from build123d import *

# Parameters (mm, degrees)
CROQUIS5_R              = 10
SALIENTE_EXTRUIR1_DEPTH = 9
CROQUIS6_R              = 14.5
SALIENTE_EXTRUIR2_DEPTH = 13
CROQUIS7_R              = 22
SALIENTE_EXTRUIR3_DEPTH = 6
CROQUIS8_R              = 12
CORTAR_EXTRUIR1_DEPTH   = 16
CROQUIS9_R              = 3
CORTAR_EXTRUIR2_DEPTH   = 16
CROQUIS10_W             = 3
CROQUIS10_H             = 9
SALIENTE_EXTRUIR4_DEPTH = 13
SALIENTE_EXTRUIR5_DEPTH = 13
CROQUIS12_W             = 8
CROQUIS12_H             = 3.8
CORTAR_EXTRUIR3_DEPTH   = 13
CROQUIS13_R             = 3
CORTAR_EXTRUIR4_DEPTH   = 13
CROQUIS14_R             = 2.05
CORTAR_EXTRUIR5_DEPTH   = 13


with BuildPart() as part:
    # Croquis5 → Saliente-Extruir1 (new body)
    with BuildSketch(Plane(origin=(0, 0, 0), x_dir=(1, 0, 0), z_dir=(0, 1, 0))):
        with Locations(Location((0, 0, 0), (0, 0, 270))):
            Circle(CROQUIS5_R)
    extrude(amount=SALIENTE_EXTRUIR1_DEPTH)

    # Croquis6 → Saliente-Extruir2 (add)
    with BuildSketch(Plane(origin=(0, 9, 0), x_dir=(1, 0, 0), z_dir=(0, 1, 0))):
        with Locations(Location((0, 0, 0), (0, 0, 90))):
            Circle(CROQUIS6_R)
    extrude(amount=SALIENTE_EXTRUIR2_DEPTH)

    # Croquis7 → Saliente-Extruir3 (add)
    with BuildSketch(Plane(origin=(0, 22, 0), x_dir=(1, 0, 0), z_dir=(0, 1, 0))):
        with Locations(Location((0, 0, 0), (0, 0, 270))):
            Circle(CROQUIS7_R)
    extrude(amount=SALIENTE_EXTRUIR3_DEPTH)

    # Croquis8 → Cortar-Extruir1 (cut)
    with BuildSketch(Plane(origin=(0, 28, 0), x_dir=(1, 0, 0), z_dir=(0, 1, 0))):
        with Locations(Location((0, 0, 0), (0, 0, 270))):
            Circle(CROQUIS8_R)
    extrude(amount=-CORTAR_EXTRUIR1_DEPTH, mode=Mode.SUBTRACT)

    # Croquis9 → Cortar-Extruir2 (cut)
    with BuildSketch(Plane(origin=(0, 12, 0), x_dir=(1, 0, 0), z_dir=(0, 1, 0))):
        with Locations(Location((0, 0, 0), (0, 0, 270))):
            Circle(CROQUIS9_R)
    extrude(amount=-CORTAR_EXTRUIR2_DEPTH, mode=Mode.SUBTRACT)

    # Croquis10 → Saliente-Extruir4 (add)
    with BuildSketch(Plane.XY):
        with Locations((0, 4.5)):
            Rectangle(CROQUIS10_W, CROQUIS10_H)
    extrude(amount=SALIENTE_EXTRUIR4_DEPTH)

    # Croquis11 → Saliente-Extruir5 (add)
    with BuildSketch(Plane.XZ):
        with BuildLine():
            Line((-1.5, 13), (1.5, 13))
            ThreePointArc((1.5, 13), (0, 14.5), (-1.5, 13))
        make_face()
    extrude(amount=-SALIENTE_EXTRUIR5_DEPTH)

    # Croquis12 → Cortar-Extruir3 (cut)
    with BuildSketch(Plane(origin=(0, 0, 0), x_dir=(0, 0, -1), z_dir=(1, 0, 0))):
        with Locations((0, 4.9)):
            Rectangle(CROQUIS12_W, CROQUIS12_H)
    extrude(amount=CORTAR_EXTRUIR3_DEPTH, mode=Mode.SUBTRACT)

    # Croquis13 → Cortar-Extruir4 (cut)
    with BuildSketch(Plane(origin=(0, 12, 0), x_dir=(1, 0, 0), z_dir=(0, 1, 0))):
        with Locations(Location((0, 0, 0), (0, 0, 270))):
            Circle(CROQUIS13_R)
    extrude(amount=-CORTAR_EXTRUIR4_DEPTH, mode=Mode.SUBTRACT)

    # Croquis14 → Cortar-Extruir5 (cut)
    with BuildSketch(Plane(origin=(0, 28, 0), x_dir=(1, 0, 0), z_dir=(0, 1, 0))):
        with Locations(Location((-17.5, 0, 0), (0, 0, 270))):
            Circle(CROQUIS14_R)
        with Locations(Location((15.999727998, 7, 0), (0, 0, 270))):
            Circle(CROQUIS14_R)
        with Locations(Location((15.999727998, -7, 0), (0, 0, 270))):
            Circle(CROQUIS14_R)
    extrude(amount=-CORTAR_EXTRUIR5_DEPTH, mode=Mode.SUBTRACT)


solid = part.part
Work out the finished part from the listing and answer in its coordinate system (mm). A direction names the side the tool comes from. Round coordinates to 2 decimals unless told otherwise and drop trailing zeros. Loops run counter-clockwise (first coordinate to the right, second up) from the corner with the lowest first, then second, coordinate; pieces in that order, holes last. Notation, with made-up numbers: (-38, -27.5) - (-6, -27.5) arc R25 ccw to (-6, -1.5) - close; hole circle Ø5 at (-40, 24.5). An arc over 180 degrees is marked (long way). One line per item, written item: value.
Q1. Find section B-B on y = 1.5. Give the vertices of the cut face in (x, z), and give its area (3 significant figures).
Check values:
outline: (-1.5, 9.89) arc R10 ccw (long way) to (1.5, 9.89) - (1.5, 13) arc R1.5 ccw to (-1.5, 13) - close; hole circle Ø6 at (0, 0)
area: 299 mm2
Q2. The mould has two halves that part along X. Classify faces 1 (the flat face through (-1.5, 4, 11)), 2 (the cylindrical face through (-21.477, 24.958, -4.769)), 3 (the cylindrical face through (-15.467, 25.042, -0.267)): +X half, -X half, draft (parallel to the pull), parting line (faces both ways), or undercut.
Check values:
face 1: -X half
face 2: parting line
face 3: undercut
Q3. Find section D-D on x = -17.5. Give the vertices of the cut face in (y, z).
Check values:
outline: (22, -13.33) - (28, -13.33) - (28, -2.05) - (22, -2.05) - close; (22, 2.05) - (28, 2.05) - (28, 13.33) - (22, 13.33) - close
Q4. Find section C-C on z = 7. Give the vertices of the cut face in (x, y).
Check values:
outline: (-20.86, 22) - (-12.7, 22) - (-12.7, 9) - (-7.14, 9) - (-7.14, 0) - (7.14, 0) - (7.14, 9) - (12.7, 9) - (12.7, 22) - (13.95, 22) - (13.95, 28) - (9.75, 28) - (9.75, 12) - (-9.75, 12) - (-9.75, 28) - (-20.86, 28) - close; (18.05, 22) - (20.86, 22) - (20.86, 28) - (18.05, 28) - close
Q5. For faces 4 (the flat face through (6, 6.8, 0)), 5 (the cylindrical face through (0, 4.4, 14.5)), 6 (the cylindrical face through (-6, 4, -8)), 7 (the flat face through (-2.5, 12, 2.5)), determine the directions among +Z, -Z, +X, -X, +Y, -Y from which every point of the face is accessible in a straight line to the end or side of a thin tool.
Check values:
face 4: +X
face 5: +Z, -Y
face 6: -Y
face 7: +Y
Q6. Find section A-A on z = 0. Give the vertices of the cut face in (x, y), and give its area (3 significant figures).
Check values:
outline: (-22, 22) - (-19.55, 22) - (-19.55, 28) - (-22, 28) - close; (-15.45, 22) - (-14.5, 22) - (-14.5, 9) - (-10, 9) - (-10, 0) - (-3, 0) - (-3, 12) - (-12, 12) - (-12, 28) - (-15.45, 28) - close; (3, 0) - (10, 0) - (10, 3) - (3, 3) - close; (3, 6.8) - (10, 6.8) - (10, 9) - (14.5, 9) - (14.5, 22) - (22, 22) - (22, 28) - (12, 28) - (12, 12) - (3, 12) - close
area: 314 mm2
Q7. Straight lines are drawn through the part: probe 1 along Y at (x, z) = (4, -1.5); probe 2 along X at (y, z) = (16.5, 0); probe 3 along Y at (x, z) = (16.5, 14). For each, find the intervals that lie inside material, in ascending order.
Check values:
probe 1: 0 to 3, 6.8 to 12
probe 2: -14.5 to -12, 12 to 14.5
probe 3: 22 to 28
Q8. Each of these flat-tipped pins is pushed along its axis until it touches: pin 1 Ø5.5 at (x, z) = (16, -7) entering from -Y; pin 2 Ø3.5 at (x, z) = (-17.5, 0) entering from -Y; pin 3 Ø8 at (y, z) = (13, 11.5) entering from -X; pin 4 Ø2.5 at (x, z) = (6.5, -1.5) entering from +Y. Where does it stop, or does it pass through?
Check values:
pin 1: y = 22
pin 2: through
pin 3: x = -12.41
pin 4: y = 12
